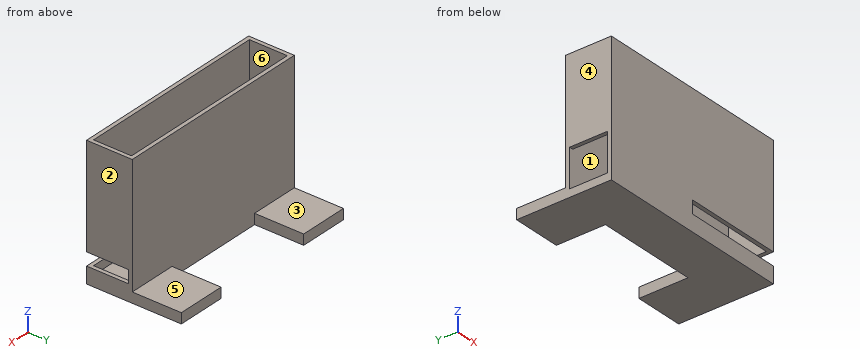
from build123d import *

# Parameters (mm, degrees)
F0_W     = 77.676
F0_H     = 17.732
F0_W_2   = 74.676
F0_H_2   = 14.732
F1_DEPTH = 50.8
F2_DEPTH = 3
F3_W     = 19.05
F3_H     = 4
F4_DEPTH = 19.05
F5_W     = 14.732
F5_H     = 14.732
F6_DEPTH = 5
F7_W     = 38.838
F7_H     = 5
F8_DEPTH = 16.232


with BuildPart() as f1:
    # F0 (on Top) → F1 (new body)
    with BuildSketch(Plane.XY):
        Rectangle(F0_W, F0_H)
        Rectangle(F0_W_2, F0_H_2, mode=Mode.SUBTRACT)
    extrude(amount=F1_DEPTH)

    # F0 (on Top) → F2 (join)
    with BuildSketch(Plane.XY):
        Rectangle(F0_W_2, F0_H_2)
    extrude(amount=F2_DEPTH)

    # F3 (on face) → F4 (join)
    with BuildSketch(Plane(origin=(0, 8.866, 0), x_dir=(-1, 0, 0), z_dir=(0, 1, 0))):
        with Locations((-29.313, 2)):
            Rectangle(F3_W, F3_H)
        with Locations((29.313, 2)):
            Rectangle(F3_W, F3_H)
    extrude(amount=F4_DEPTH)

    # F5 (on face) → F6 (cut)
    with BuildSketch(Plane(origin=(-38.838, 0, 0), x_dir=(0, -1, 0), z_dir=(-1, 0, 0))):
        with Locations((0, 10.366)):
            Rectangle(F5_W, F5_H)
    extrude(amount=-F6_DEPTH, mode=Mode.SUBTRACT)

    # F7 (on face) → F8 (cut)
    with BuildSketch(Plane.XZ.offset(8.866)):
        with Locations((19.419, 8.85)):
            Rectangle(F7_W, F7_H)
    extrude(amount=-F8_DEPTH, mode=Mode.SUBTRACT)


solid = f1.part
Read the model definition and answer for the solid it produces. Units are mm, in the model's axes. Face numbers are marked on the shaded views. A direction names the side the tool comes from. Give positions to 0.01 mm unless a question says otherwise; leave off trailing zeros. Loops run counter-clockwise (first coordinate to the right, second up) from the corner with the lowest first, then second, coordinate; pieces in that order, holes last. Notation, with made-up numbers: (51.5, 8) - (93.5, 8) arc R26 cw to (93.5, 30) - close; hole circle Ø4 at (4.5, 53.25). An arc over 180 degrees is marked (long way). Answer as CSV lines item,"result". Start each with the question number.
1) Straight lines are drawn through the part: L1, parallel to Y at x = -3.5, z = 7; L2, parallel to X at y = -4, z = 38.5; L3, parallel to Z at x = -1.5, y = 5.5. For each, find the intervals that lie inside material, in ascending order. Write a range as from..to.
2) Determine the mould class of the marked faces 1, 2 and 3 for opening direction X: released by +X, released by -X, zero draft, split by the parting line, or undercut.
3) Which of the six approach directions +Z, -Z, +X, -X, +Y, -Y give full straight-line access (tool end or side, diameter ignored) to the marked faces 4, 5 and 6?
4) Find section A-A (x = 32.5). Write down the section's boundary in (y, z).
5) Find section C-C (z = 8). Write down the section's boundary in (x, y).
6) Find section B-B (y = -0.5). Write down the section's boundary in (x, z), then the cut area to 3 significant figures.
7) Each of these flat-tipped pins is pushed along its axis until it touches: pin 1 Ø18 at (x, y) = (18, 0.5) entering from -Z; pin 2 Ø5.5 at (x, y) = (-33.5, 14) entering from +Z; pin 3 Ø1 at (y, z) = (0.5, 4.5) entering from -X; pin 4 Ø8 at (y, z) = (18.5, 11) entering from -X. Where does it stop, or does it pass through?
8) Find section D-D (z = 37). Write down the section's boundary in (x, y), then the cut area to 3 significant figures.
Findings below:
1,L1,"-8.87..-7.37, 7.37..8.87"
1,L2,"-38.84..-37.34, 37.34..38.84"
1,L3,"0..3"
2,face 1,"undercut"
2,face 2,"released by +X"
2,face 3,"zero draft"
3,face 4,"+Z, -Z, -X, +Y, -Y"
3,face 5,"+Z, +X, -X, +Y"
3,face 6,"+Z"
4,outline,"(-8.87, 0) - (27.92, 0) - (27.92, 4) - (8.87, 4) - (8.87, 50.8) - (7.37, 50.8) - (7.37, 3) - (-7.37, 3) - (-7.37, 6.35) - (-8.87, 6.35) - close; (-8.87, 11.35) - (-7.37, 11.35) - (-7.37, 50.8) - (-8.87, 50.8) - close"
5,outline,"(-38.84, -8.87) - (0, -8.87) - (0, -7.37) - (-38.84, -7.37) - close; (-38.84, 7.37) - (38.84, 7.37) - (38.84, 8.87) - (-38.84, 8.87) - close"
6,outline,"(-38.84, 0) - (38.84, 0) - (38.84, 6.35) - (37.34, 6.35) - (37.34, 3) - (-38.84, 3) - close; (-38.84, 17.73) - (-37.34, 17.73) - (-37.34, 50.8) - (-38.84, 50.8) - close; (37.34, 11.35) - (38.84, 11.35) - (38.84, 50.8) - (37.34, 50.8) - close"
6,area,"347 mm^2"
7,pin 1,"z = 0"
7,pin 2,"z = 4"
7,pin 3,"x = 37.34"
7,pin 4,"through"
8,outline,"(-38.84, -8.87) - (38.84, -8.87) - (38.84, 8.87) - (-38.84, 8.87) - close; hole (-37.34, -7.37) - (37.34, -7.37) - (37.34, 7.37) - (-37.34, 7.37) - close"
8,area,"277 mm^2"
